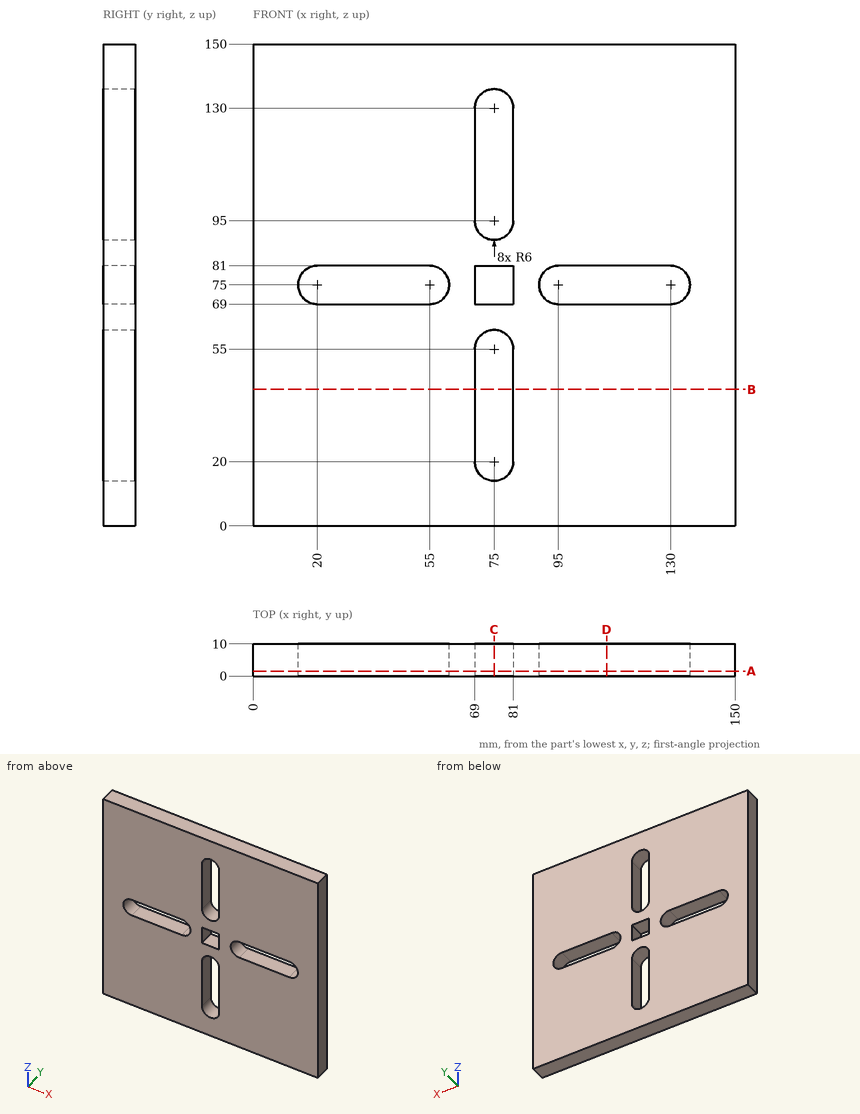
Part print with two shaded views. Sizes in mm from the minimum x, y, z corner. Give positions to 0.01 mm unless a question says otherwise; leave off trailing zeros. Order: outer loops, then holes, each group sorted by start corner. A loop starts at its lowest first (then second) coordinate and runs counter-clockwise, first axis right, second up.
(1) Saw through at A-A, the plane y = 1.5. Give the cut face in (x, z), then the cut area to 3 significant figures.
(2) Drill centre lines: L1, parallel to X at y = 0.5, z = 113.5; L2, parallel to X at y = 4.25, z = 77. Where is each one in solid material? Low to high.
(3) Flat gauge pin, fed straight in: pin 1 (3 mm diameter, centred on y = 7, z = 44, fed in from -X). Where does the tip first touch, or does it go through?
(4) Saw through at D-D, the plane x = 110. Give the cut face in (y, z).
(5) Saw through at C-C, the plane x = 75. Give the cut face in (y, z).
(6) Saw through at B-B, the plane z = 42.5. Give the cut face in (x, y).
Results found:
1. outline: (0, 0) - (150, 0) - (150, 150) - (0, 150) - close; hole (20, 69) - (55, 69) arc R6 ccw to (55, 81) - (20, 81) arc R6 ccw to start; hole (69, 20) arc R6 ccw to (81, 20) - (81, 55) arc R6 ccw to (69, 55) - close; hole (69, 69) - (81, 69) - (81, 81) - (69, 81) - close; hole (69, 95) arc R6 ccw to (81, 95) - (81, 130) arc R6 ccw to (69, 130) - close; hole (95, 69) - (130, 69) arc R6 ccw to (130, 81) - (95, 81) arc R6 ccw to start
1. area: 20,200 mm2
2. L1: x = 0 to 69, 81 to 150
2. L2: x = 0 to 14.34, 60.66 to 69, 81 to 89.34, 135.66 to 150
3. pin 1: stops at x = 0
4. outline: (0, 0) - (10, 0) - (10, 69) - (0, 69) - close; (0, 81) - (10, 81) - (10, 150) - (0, 150) - close
5. outline: (0, 0) - (10, 0) - (10, 14) - (0, 14) - close; (0, 61) - (10, 61) - (10, 69) - (0, 69) - close; (0, 81) - (10, 81) - (10, 89) - (0, 89) - close; (0, 136) - (10, 136) - (10, 150) - (0, 150) - close
6. outline: (0, 0) - (69, 0) - (69, 10) - (0, 10) - close; (81, 0) - (150, 0) - (150, 10) - (81, 10) - close
